Design review of the part built by this model. Coordinates are the model's own, in mm. Face numbers are marked on the shaded views. A direction names the side the tool comes from. Round coordinates to 2 decimals unless told otherwise and drop trailing zeros. Order: outer loops, then holes, each group sorted by start corner. A loop starts at its lowest first (then second) coordinate and runs counter-clockwise, first axis right, second up. Notation, with made-up numbers: (-8.75, 86.5) - (27.25, 86.5) arc R16 cw to (27.25, 114.5) - close; hole circle Ø2 at (-22.5, 54.25). An arc over 180 degrees is marked (long way). Answer as a JSON object with one key per item and string values. Group by question number.
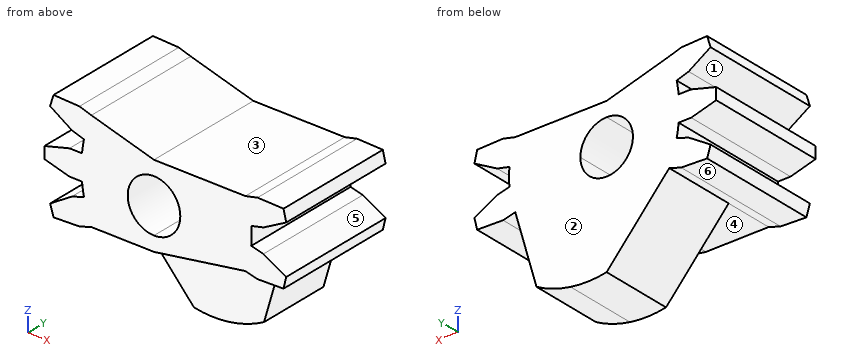
from build123d import *

# Parameters (mm, degrees)
BOSS_EXTRUDE1_DEPTH = 9.7
BOSS_EXTRUDE2_DEPTH = 5.8
CUT_EXTRUDE1_DEPTH  = 15.880557968
BOSS_EXTRUDE3_REACH = 16.881
CUT_EXTRUDE2_DEPTH  = 17.567792011
BOSS_EXTRUDE4_START = -9.7
BOSS_EXTRUDE4_DEPTH = 9.7
BOSS_EXTRUDE5_DEPTH = 5.8


# Read off the part's stored shape, not the designer's step: Boss-Extrude4
with BuildPart() as part:
    # Sketch1 → Boss-Extrude1 (new body)
    with BuildSketch(Plane(origin=(0, 0, 0), x_dir=(1, 0, 0), z_dir=(0, 1, 0))):
        Polygon((6.15, 2.65), (6.15, -2.65), (-1.15, -2.65), (-6.15, -4.038578044), (-6.15, 3.861421956), (-1.15, 3.861421956), align=None)
    extrude(amount=BOSS_EXTRUDE1_DEPTH)

    # Sketch2 → Boss-Extrude2 (add)
    with BuildSketch(Plane.XZ):
        Polygon((-6.15, -3.861421956), (-1.15, -9.461421956), (-1.15, -3.861421956), align=None)
        Polygon((-1.15, -3.861421956), (-1.15, -9.461421956), (4.45, -8.532111962), (4.45, -2.932111962), align=None)
        Polygon((4.45, -2.932111962), (4.45, -8.532111962), (6.15, -2.65), align=None)
    extrude(amount=-BOSS_EXTRUDE2_DEPTH)

    # Sketch3 → Cut-Extrude1 (cut, through all)
    with BuildSketch(Plane(origin=(0, 9.7, 0), x_dir=(1, 0, 0), z_dir=(0, 1, 0))):
        with BuildLine():
            ThreePointArc((0.95, 0.605710978), (0.33492424, 2.090635219), (-1.15, 2.705710978))
            Line((-1.15, 2.705710978), (-1.15, -1.494289022))
            ThreePointArc((-1.15, -1.494289022), (0.33492424, -0.879213262), (0.95, 0.605710978))
        make_face()
        with BuildLine():
            Line((-1.15, -1.494289022), (-1.15, 2.705710978))
            ThreePointArc((-1.15, 2.705710978), (-3.25, 0.605710978), (-1.15, -1.494289022))
        make_face()
    extrude(amount=-CUT_EXTRUDE1_DEPTH, mode=Mode.SUBTRACT)

    # Boss-Extrude3: up to this face of the body (flat: up to its plane)
    boss_extrude3_end = Plane(part.part.faces().sort_by_distance((0.174384558, 0, -2.694350329))[0])
    # Sketch4 → Boss-Extrude3 (add, up to the picked face)
    with BuildSketch(Plane(origin=(0, 9.7, 0), x_dir=(1, 0, 0), z_dir=(0, 1, 0)), mode=Mode.PRIVATE) as boss_extrude3_sk1:
        with BuildLine():
            Line((6.615749123, 0.704986439), (9.533269465, 1.403610124))
            Line((9.533269465, 1.403610124), (9.067520342, 3.348623685))
            Line((9.067520342, 3.348623685), (6.15, 2.65))
            Line((6.15, 2.65), (6.15, -2.65))
            Line((6.15, -2.65), (9.067520342, -3.348623685))
            Line((9.067520342, -3.348623685), (9.533269465, -1.403610124))
            Line((9.533269465, -1.403610124), (6.615749123, -0.704986439))
            ThreePointArc((6.615749123, -0.704986439), (6.65, 0), (6.615749123, 0.704986439))
        make_face()
    boss_extrude3_tool1 = split(extrude(boss_extrude3_sk1.sketch, amount=-BOSS_EXTRUDE3_REACH, mode=Mode.PRIVATE), bisect_by=boss_extrude3_end, keep=Keep.BOTH, mode=Mode.PRIVATE)
    add(boss_extrude3_tool1.solids().sort_by(Axis((6.574967, 9.7, 0), (0, -1, 0)))[0])

    # Sketch5 → Cut-Extrude2 (cut, through all)
    with BuildSketch(Plane(origin=(0, 9.7, 0), x_dir=(1, 0, 0), z_dir=(0, 1, 0))):
        Polygon((9.067520342, 3.348623685), (7.122506781, 2.882874562), (9.192317444, 2.827458872), align=None)
        Polygon((9.408472364, 1.924774937), (7.588255904, 0.937861), (9.533269465, 1.403610124), align=None)
        Polygon((9.408472364, -1.924774937), (9.533269465, -1.403610124), (7.588255904, -0.937861), align=None)
        Polygon((9.192317444, -2.827458872), (7.122506781, -2.882874562), (9.067520342, -3.348623685), align=None)
    extrude(amount=-CUT_EXTRUDE2_DEPTH, mode=Mode.SUBTRACT)

    # Boss-Extrude4 outline → Boss-Extrude4 (add)
    with BuildSketch(Plane(origin=(0, 9.7, 0), x_dir=(1, 0, 0), z_dir=(0, 1, 0)).offset(BOSS_EXTRUDE4_START)):
        with BuildLine():
            Line((-6.900626431, 0.911421956), (-7.900631816, 0.911421956))
            Line((-7.900631816, 0.911421956), (-9.900626719, 0.375520635))
            Line((-9.900626719, 0.375520635), (-9.900626431, -0.552684328))
            Line((-9.900626431, -0.552684328), (-7.900627802, -1.088578044))
            Line((-7.900627802, -1.088578044), (-6.900626431, -1.088578044))
            ThreePointArc((-6.900626431, -1.088578044), (-6.835256527, -1.610578376), (-6.742932214, -2.128491295))
            Line((-6.742932214, -2.128491295), (-7.697979422, -2.424958592))
            Line((-7.697979422, -2.424958592), (-9.449184507, -3.529703076))
            Line((-9.449184507, -3.529703076), (-9.1740036, -4.416177353))
            Line((-9.1740036, -4.416177353), (-7.105039542, -4.335042961))
            Line((-7.105039542, -4.335042961), (-6.15, -4.038578044))
            Line((-6.15, -4.038578044), (-6.15, 3.861421956))
            Line((-6.15, 3.861421956), (-7.105043375, 4.157888063))
            Line((-7.105043375, 4.157888063), (-9.174005832, 4.239014076))
            Line((-9.174005832, 4.239014076), (-9.44918663, 3.35253973))
            Line((-9.44918663, 3.35253973), (-7.697975589, 2.247801314))
            Line((-7.697975589, 2.247801314), (-6.742932214, 1.951335207))
            ThreePointArc((-6.742932214, 1.951335207), (-6.835256527, 1.433422288), (-6.900626431, 0.911421956))
        make_face()
    extrude(amount=BOSS_EXTRUDE4_DEPTH)

    # Sketch8 → Boss-Extrude5 (add)
    with BuildSketch(Plane(origin=(0, 5.8, 0), x_dir=(1, 0, 0), z_dir=(0, 1, 0))):
        with BuildLine():
            ThreePointArc((1.731854671, 9.490021268), (0.289677429, 9.601670434), (-1.15, 9.461421956))
            Line((-1.15, 9.461421956), (1.65, 8.996766959))
            Line((1.65, 8.996766959), (1.731854671, 9.490021268))
        make_face()
        with BuildLine():
            Line((1.731854671, 9.490021268), (1.65, 8.996766959))
            Line((1.65, 8.996766959), (4.45, 8.532111962))
            ThreePointArc((4.45, 8.532111962), (3.132791885, 9.12986067), (1.731854671, 9.490021268))
        make_face()
    extrude(amount=-BOSS_EXTRUDE5_DEPTH)


with BuildPart() as body_2:
    # Mirror1: mirrored copy
    add(part.part.mirror(Plane.ZX))


solid = body_2.part
1. Take a section at C-C, the plane z = -7.5. Give the boundary of the cut face in (x, y), then the cut area to 3 significant figures.
2. To check wall thickness, follow line 1 (Z direction, x = -7.5, y = -1); line 2 (Z direction, x = -8.5, y = -5); line 3 (Y direction, x = 6, z = -3). State the ranges of each line that lie inside material, in increasing order. Write a range as from..to.
3. Take a section at B-B, the plane x = 5.25. Give the boundary of the cut face in (y, z).
4. Take a section at A-A, the plane x = 0.25. Give the boundary of the cut face in (y, z).
5. Tool access review of the marked faces 4, 5 and 6: name each direction out of +Z, -Z, +X, -X, +Y, -Y from which nothing blocks a thin tool from reaching the whole face with its end or side.
6. Mouldability with a two-part tool opening along Z and no side actions: class the marked faces 1, 2 and 3 as pulls with the +Z half, pulls with the -Z half, needs draft (parallel to the pull), parting line crosses it, or undercut.
7. Clearance check with flat-ended pins moving along their axes: P1, Ø0.8, axis at x = -7, y = -6.5, coming from the -Z side; P2, Ø1, axis at y = -8, z = -2, coming from the -X side; P3, Ø4, axis at x = -7, z = -6.5, coming from the +Y side; P4, Ø1, axis at y = -1, z = -3.5, coming from the +X side. State where each tip first meets the part, or that it passes through.
8. Take a section at D-D, the plane x = 2.5. Give the boundary of the cut face in (y, z).
Response values:
{
 "1": {"outline": "(-2.9, -5.8) - (4.75, -5.8) - (4.75, 0) - (-2.9, 0) - close", "area": "44.4 mm2"},
 "2": {"line 1": "-4.17..-2.19, -0.91..1.09, 2.36..4.35", "line 2": "-4.21..-2.75, -0.75..0.93, 2.93..4.39", "line 3": "-5.8..0"},
 "3": {"outline": "(-9.7, -2.8) - (-5.8, -2.8) - (-5.8, -5.76) - (0, -5.76) - (0, 2.65) - (-9.7, 2.65) - close"},
 "4": {"outline": "(-9.7, -3.63) - (-5.8, -3.63) - (-5.8, -9.6) - (0, -9.6) - (0, -2.17) - (-9.7, -2.17) - close; (-9.7, 0.96) - (0, 0.96) - (0, 2.65) - (-9.7, 2.65) - close"},
 "5": {"face 4": "-Z, +X, -Y", "face 5": "+X, +Y, -Y", "face 6": "-Z, +Y, -Y"},
 "6": {"face 1": "undercut", "face 2": "needs draft", "face 3": "pulls with the +Z half"},
 "7": {"P1": "z = -4.17", "P2": "x = -8.1", "P3": "through", "P4": "x = 6.05"},
 "8": {"outline": "(-9.7, -3.26) - (-5.8, -3.26) - (-5.8, -9.32) - (0, -9.32) - (0, 2.65) - (-9.7, 2.65) - close"}
}
